Read the model definition and answer for the solid it produces. Units are mm, in the model's axes. A direction names the side the tool comes from. Coordinates: 2 decimals unless noted, no trailing zeros. Write each loop counter-clockwise with the first axis right and the second up, starting at its lowest first coordinate (ties: lowest second). Pieces come first, ordered by that corner, then holes. Notation, with made-up numbers: (40.5, -14.75) -> (61.5, -14.75) arc R24 cw to (61.5, 23.25) -> close; hole circle Ø7 at (4, 27). An arc over 180 degrees is marked (long way). Answer in a Markdown table with one row per item. Add a question column.
Item 1: Which of the six approach directions +Z, -Z, +X, -X, +Y, -Y give full straight-line access (tool end or side, diameter ignored) to faces 1 (the face through (-13, -5.83, 3)), 2 (the face through (4, -3, 1)), 3 (the face through (-13, -2.53, 3))?
Item 2: Straight lines are drawn through the part: line 1 (X direction, y = -4, z = 3.45); line 2 (X direction, y = -3.1, z = 1.2); line 3 (Z direction, x = -1.5, y = -6.2). For each, find the intervals that lie inside material, in ascending order. Write a range as from..to.
Item 3: Section C-C on x = 4 is taken. Write down the section's boundary in (y, z).
Item 4: Section A-A on z = 2.75 is taken. Write down the section's boundary in (x, y).
Item 5: Section B-B on x = -14 is taken. Write down the section's boundary in (y, z).
Item 6: For a pull along X with two mould halves and no side action, classify faces 4 (the face through (26.3, -4.2, 2.6)), 5 (the face through (14.9, -4.2, 2.6)), 6 (the face through (-2, -4, 4.5)) as +X half, -X half, draft (parallel to the pull), parting line (faces both ways), or undercut.
Item 7: Given pin 1 Ø1.6 at (x, z) = (21.5, 3) entering from -Y; pin 2 Ø1.5 at (y, z) = (-5.5, 3) entering from +X; pin 3 Ø1 at (x, z) = (-2, 2) entering from +Y, each flat-ended and moving along its own axis, determine where each tip first touches the part or whether it passes through.
```python
from build123d import *

# Parameters (mm, degrees)
F0_W     = 45.4
F0_H     = 5
F1_DEPTH = 1
F2_W     = 6.8
F2_H     = 3.3
F3_DEPTH = 3.5
F4_R     = 1
F5_R     = 0.3


with BuildPart() as f1:
    # F0 (on Top) → F1 (new body)
    with BuildSketch(Plane.XY):
        with Locations((4.700655, -4.029623)):
            Rectangle(F0_W, F0_H)
    extrude(amount=F1_DEPTH)

    # F2 (on face) → F3 (join)
    with BuildSketch(Plane.XY.offset(1)):
        with Locations((-12.949345, -4.179623)):
            Rectangle(F2_W, F2_H)
        with BuildLine():
            Line((-16.349345, -5.829623), (-16.349345, -2.529623))
            ThreePointArc((-16.349345, -2.529623), (-17.999345, -4.179623), (-16.349345, -5.829623))
        make_face()
        with BuildLine():
            ThreePointArc((-9.549345, -5.829623), (-7.899345, -4.179623), (-9.549345, -2.529623))
            Line((-9.549345, -2.529623), (-9.549345, -5.829623))
        make_face()
        with BuildLine():
            Line((-4.949345, -5.829623), (-4.949345, -2.529623))
            ThreePointArc((-4.949345, -2.529623), (-6.599345, -4.179623), (-4.949345, -5.829623))
        make_face()
        with Locations((-1.549345, -4.179623)):
            Rectangle(F2_W, F2_H)
        with BuildLine():
            ThreePointArc((1.850655, -5.829623), (3.500655, -4.179623), (1.850655, -2.529623))
            Line((1.850655, -2.529623), (1.850655, -5.829623))
        make_face()
        with BuildLine():
            Line((6.450655, -5.829623), (6.450655, -2.529623))
            ThreePointArc((6.450655, -2.529623), (4.800655, -4.179623), (6.450655, -5.829623))
        make_face()
        with Locations((9.850655, -4.179623)):
            Rectangle(F2_W, F2_H)
        with BuildLine():
            ThreePointArc((13.250655, -5.829623), (14.900655, -4.179623), (13.250655, -2.529623))
            Line((13.250655, -2.529623), (13.250655, -5.829623))
        make_face()
        with BuildLine():
            Line((17.850655, -5.829623), (17.850655, -2.529623))
            ThreePointArc((17.850655, -2.529623), (16.200655, -4.179623), (17.850655, -5.829623))
        make_face()
        with Locations((21.250655, -4.179623)):
            Rectangle(F2_W, F2_H)
        with BuildLine():
            ThreePointArc((24.650655, -5.829623), (26.300655, -4.179623), (24.650655, -2.529623))
            Line((24.650655, -2.529623), (24.650655, -5.829623))
        make_face()
    extrude(amount=F3_DEPTH)

    # F4
    f4_edges = [f1.edges().sort_by_distance(p)[0] for p in [
        (-17.999345, -1.529623, 0.5),
        (-17.999345, -6.529623, 0.5),
        (27.400655, -1.529623, 0.5),
        (27.400655, -6.529623, 0.5),
    ]]
    fillet(f4_edges, radius=F4_R)

    # F5
    f5_edges = [f1.edges().sort_by_distance(p)[0] for p in [
        (-17.999345, -4.179623, 4.5),
        (-6.599345, -4.179623, 4.5),
        (4.800655, -4.179623, 4.5),
        (16.200655, -4.179623, 4.5),
    ]]
    fillet(f5_edges, radius=F5_R)


solid = f1.part
```
Results below:
| question | item | result |
|---|---|---|
| 1 | face 1 | +Z, +X, -X, -Y |
| 1 | face 2 | +Z |
| 1 | face 3 | +Z, +X, -X, +Y |
| 2 | line 1 | x = -17.99..-7.91, -6.59..3.49, 4.81..14.89, 16.21..26.29 |
| 2 | line 2 | x = -17.6..-8.3, -6.2..3.1, 5.2..14.5, 16.6..25.9 |
| 2 | line 3 | z = 0..1 |
| 3 | outline | (-6.53, 0) -> (-1.53, 0) -> (-1.53, 1) -> (-6.53, 1) -> close |
| 4 | outline | (-16.35, -5.83) -> (-9.55, -5.83) arc R1.65 ccw to (-9.55, -2.53) -> (-16.35, -2.53) arc R1.65 ccw to start; (-4.95, -5.83) -> (1.85, -5.83) arc R1.65 ccw to (1.85, -2.53) -> (-4.95, -2.53) arc R1.65 ccw to start; (6.45, -5.83) -> (13.25, -5.83) arc R1.65 ccw to (13.25, -2.53) -> (6.45, -2.53) arc R1.65 ccw to start; (17.85, -5.83) -> (24.65, -5.83) arc R1.65 ccw to (24.65, -2.53) -> (17.85, -2.53) arc R1.65 ccw to start |
| 5 | outline | (-6.53, 0) -> (-1.53, 0) -> (-1.53, 1) -> (-2.53, 1) -> (-2.53, 4.2) arc R0.3 ccw to (-2.83, 4.5) -> (-5.53, 4.5) arc R0.3 ccw to (-5.83, 4.2) -> (-5.83, 1) -> (-6.53, 1) -> close |
| 6 | face 4 | +X half |
| 6 | face 5 | undercut |
| 6 | face 6 | draft |
| 7 | pin 1 | stops at y = -5.83 |
| 7 | pin 2 | stops at x = 26.2 |
| 7 | pin 3 | stops at y = -2.53 |
